Check sheet for the drawn part. Datum: minimum x, y, z corner. Units: mm. A direction names the side the tool comes from. Round coordinates to 2 decimals unless told otherwise and drop trailing zeros. Write each loop counter-clockwise with the first axis right and the second up, starting at its lowest first coordinate (ties: lowest second). Pieces come first, ordered by that corner, then holes. Notation, with made-up numbers: (65, 3.25) -> (109, 3.25) arc R25 cw to (109, 20.25) -> close; hole circle Ø6 at (4, -2). An arc over 180 degrees is marked (long way). One line per item, written item: value.
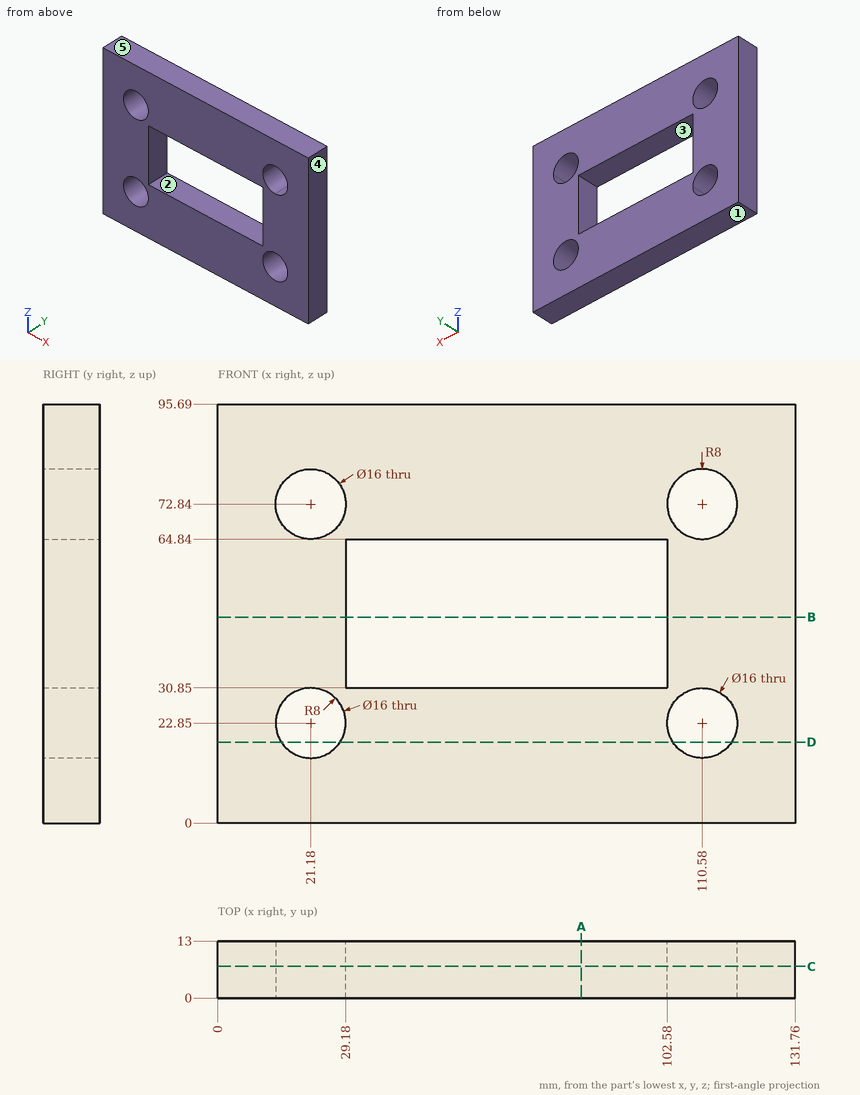
Item 1: Mould release check, pull along X, two halves, no side actions. Record for the marked faces 3, 4 and 5: pulls with the +X half, pulls with the -X half, needs draft (parallel to the pull), parting line crosses it, or undercut.
Answer:
face 3: undercut
face 4: pulls with the +X half
face 5: needs draft
Item 2: Sectioned sample at C-C on y = 7.25. Enter the section's corners in (x, z), and give its area (3 significant figures).
Answer:
outline: (0, 0) -> (131.76, 0) -> (131.76, 95.69) -> (0, 95.69) -> close; hole circle Ø16 at (21.18, 22.85); hole circle Ø16 at (21.18, 72.84); hole (29.18, 30.85) -> (102.58, 30.85) -> (102.58, 64.84) -> (29.18, 64.84) -> close; hole circle Ø16 at (110.58, 22.85); hole circle Ø16 at (110.58, 72.84)
area: 9,310 mm^2
Item 3: Tool access check on the marked faces 1 and 2. Record the directions out of +Z, -Z, +X, -X, +Y, -Y that give a thin tool (end or side, any length) a straight path to the whole face; none if there is none.
Answer:
face 1: -Z, +X, -X, +Y, -Y
face 2: +Y, -Y
Item 4: Sectioned sample at B-B on z = 47. Enter the section's corners in (x, y).
Answer:
outline: (0, 0) -> (29.18, 0) -> (29.18, 13) -> (0, 13) -> close; (102.58, 0) -> (131.76, 0) -> (131.76, 13) -> (102.58, 13) -> close
Item 5: Thickness scan on line 1 (X direction, y = 4.75, z = 72.84); line 2 (X direction, y = 2.25, z = 49.5); line 3 (Z direction, x = 63, y = 5.25). Record the ranges inside material, lowest first.
Answer:
line 1: x = 0 to 13.18, 29.18 to 102.58, 118.58 to 131.76
line 2: x = 0 to 29.18, 102.58 to 131.76
line 3: z = 0 to 30.85, 64.84 to 95.69
Item 6: Sectioned sample at D-D on z = 18.5. Enter the section's corners in (x, y).
Answer:
outline: (0, 0) -> (14.47, 0) -> (14.47, 13) -> (0, 13) -> close; (27.89, 0) -> (103.87, 0) -> (103.87, 13) -> (27.89, 13) -> close; (117.29, 0) -> (131.76, 0) -> (131.76, 13) -> (117.29, 13) -> close
Item 7: Sectioned sample at A-A on x = 83. Enter the section's corners in (y, z).
Answer:
outline: (0, 0) -> (13, 0) -> (13, 30.85) -> (0, 30.85) -> close; (0, 64.84) -> (13, 64.84) -> (13, 95.69) -> (0, 95.69) -> close
